Autodesk Inventor part; units mm, degrees
ref_plane "YZ Plane" through (0, 0, 0) normal (1, 0, 0) x (0, 1, 0)
ref_plane "XZ Plane" through (0, 0, 0) normal (0, 1, 0) x (-1, 0, 0)
ref_plane "XY Plane" through (0, 0, 0) normal (0, 0, 1) x (1, 0, 0)
sketch "Sketch1" plane through (0, 0, 0) normal (0, 0, 1) x (1, 0, 0)
  line L0 (0, 0) -> (18, 0)
  line L1 (0, 0) -> (0, 9)
  line L2 (0, 9) -> (18, 9)
  line L3 (18, 9) -> (18, 0)
  dimension "d2" = 18
revolve "Revolution1" add sketch "Sketch1" angle 360 about axis through (0, 0, 0) along (1, 0, 0)
sketch "Sketch2" plane through (0, 0, 0) normal (-1, 0, 0) x (0, 0, 1)
  circle A0 centre (0, 0) radius 8
  circle A1 centre (0, 0) radius 9
  dimension "d4" = 18
  dimension "d5" = 16
hole "Hole1" at (0, 0, 0) direction (1, 0, 0) diameter 16 end through all
sketch "Sketch3" plane through (18, 0, 0) normal (1, 0, 0) x (0, 0, -1)
  circle A0 centre (0, 0) radius 9
  circle A1 centre (0, 0) radius 9
  dimension "d13" = 18
  dimension "d14" = 18
extrude "Extrusion1" add sketch "Sketch3" along normal blind 3
sketch "Sketch4" plane through (0, 0, 0) normal (-1, 0, 0) x (0, 0, 1)
  circle A0 centre (0, 0) radius 9
  circle A1 centre (0, 0) radius 8
  circle A2 centre (0, 0) radius 8.5
  line L0 (0.75, -8.75) -> (-0.75, -8.75)
  line L1 (-0.75, -8.75) -> (-0.75, -8.25)
  line L2 (-0.75, -8.25) -> (0.75, -8.25)
  line L3 (0.75, -8.25) -> (0.75, -8.75)
  line L4 (8.25, -0.75) -> (8.25, 0.75)
  line L5 (8.75, -0.75) -> (8.25, -0.75)
  line L6 (8.75, 0.75) -> (8.75, -0.75)
  line L7 (8.25, 0.75) -> (8.75, 0.75)
  line L8 (0.75, 8.25) -> (-0.75, 8.25)
  line L9 (0.75, 8.75) -> (0.75, 8.25)
  line L10 (-0.75, 8.75) -> (0.75, 8.75)
  line L11 (-0.75, 8.25) -> (-0.75, 8.75)
  line L12 (-8.25, 0.75) -> (-8.25, -0.75)
  line L13 (-8.75, 0.75) -> (-8.25, 0.75)
  line L14 (-8.75, -0.75) -> (-8.75, 0.75)
  line L15 (-8.25, -0.75) -> (-8.75, -0.75)
  dimension "d17" = 18
  dimension "d18" = 17
  dimension "d19" = 0.5
  dimension "d20" = 1.5
  dimension "d21" = 0.25
  dimension "d22" = 0.75
  dimension "d26" = 360
extrude "Extrusion2" cut sketch "Sketch4" against normal blind 2 contours A2 L5 L4 L7 | A2 L7 L6 L5 | L9 L8 L11 A2 | A2 L11 L10 L9 | L3 L0 L1 A2 | A2 L1 L2 L3 | L13 L12 L15 A2 | A2 L15 L14 L13
equation "\"d6\" = d5"
equation "\"d13\" = d14"
properties part number "McCrea_dolny_kos_walle_MIR2" material "ABS Plastic"
Source: CAD feature listing. Evaluate the final solid. Frame: model axes, mm. Round coordinates to 2 decimals unless told otherwise and drop trailing zeros. Loops run counter-clockwise (first coordinate to the right, second up) from the corner with the lowest first, then second, coordinate; pieces in that order, holes last. Notation, with made-up numbers: (-9, 49.25) - (15, 49.25) arc R20 cw to (15, 71.25) - close; hole circle Ø4 at (-21.75, 20). An arc over 180 degrees is marked (long way). Write item = value, one per line. Start each with the question number.
Item 1: Section query C-C on x = 4.25. Output: boundary loops of the cut face in (y, z), plus the area to 3 significant figures.
Item 2: First-contact query: pin 1 Ø1.5 at (x, y) = (15.5, 2.5) entering from +Z; pin 2 Ø4 at (y, z) = (0.5, -2.5) entering from -X; pin 3 Ø3 at (x, z) = (16, -3.5) entering from -Y. Flat tips, straight axial feed; report the tip coordinate or a pass-through.
Item 3: Mould query, pull axis Z, two halves, no side actions, for faces 1 (the face through (1, 0, -8.25)), 2 (the face through (9.13, 7.81, -1.73)), 3 (the face through (21, 0, 0)). Classes: released by +Z, released by -Z, zero draft, split by the parting line, or undercut.
Item 4: Section query A-A on z = 0. Output: boundary loops of the cut face in (x, y).
Item 5: Section query D-D on x = 19.75. Output: boundary loops of the cut face in (y, z).
Item 6: Material intervals for line 1 (Z direction, x = 14.25, y = 0); line 2 (X direction, y = -6.25, z = -0.75), sorted ascending.
Results list:
q1.outline = circle Ø18 at (0, 0); hole circle Ø16 at (0, 0)
q1.area = 53.4 mm²
q2.pin_1 = 8.83
q2.pin_2 = 18
q2.pin_3 = -8.77
q3.face_1 = undercut
q3.face_2 = undercut
q3.face_3 = zero draft
q4.outline = (0, -9) - (21, -9) - (21, 9) - (0, 9) - (0, 8.75) - (2, 8.75) - (2, 8.25) - (0, 8.25) - (0, 8) - (18, 8) - (18, -8) - (0, -8) - (0, -8.25) - (2, -8.25) - (2, -8.75) - (0, -8.75) - close
q5.outline = circle Ø18 at (0, 0)
q6.line_1 = -9 to -8, 8 to 9
q6.line_2 = 18 to 21
